Geometry: final body of the model. Coordinates: model frame, mm. A direction names the side the tool comes from. Give positions to 0.01 mm unless a question says otherwise; leave off trailing zeros. Loops run counter-clockwise (first coordinate to the right, second up) from the corner with the lowest first, then second, coordinate; pieces in that order, holes last. Notation, with made-up numbers: (6, 29.5) - (38, 29.5) arc R30 ccw to (38, 66.5) - close; hole circle Ø1 at (-22.5, 44). An arc over 180 degrees is marked (long way). Use CSV: the item, a comma, the result in double quotes. Start each with the question number.
```python
from build123d import *

# Parameters (mm, degrees)
SKETCH1_R            = 32.5
SKETCH1_R_2          = 17
BOSS_EXTRUDE1_DEPTH  = 6
SKETCH2_R            = 1.6
CUT_EXTRUDE1_DEPTH   = 6
LPATTERN1_COUNT      = 2
LPATTERN1_PITCH      = 36.8
LPATTERN1_COUNT_DIR2 = 2
LPATTERN1_PITCH_DIR2 = 36.8
SKETCH3_R            = 1.65
CUT_EXTRUDE2_DEPTH   = 10
CIRPATTERN1_COUNT    = 6
SKETCH6_W            = 10
SKETCH6_H            = 20
CUT_EXTRUDE4_DEPTH   = 10
SKETCH7_R            = 1.6
SKETCH7_R_2          = 1.5
CUT_EXTRUDE5_DEPTH   = 20
FILLET1_R            = 3.175
CUT_EXTRUDE6_START   = 3.1
SKETCH8_R            = 6
CUT_EXTRUDE6_DEPTH   = 20


with BuildPart() as part:
    # Sketch1 → Boss-Extrude1 (new body)
    with BuildSketch(Plane(origin=(0, 0, 0), x_dir=(1, 0, 0), z_dir=(0, 1, 0))):
        with BuildLine():
            Line((-42.5, -73.411966665), (-41.810700901, -77.192472856))
            ThreePointArc((-41.810700901, -77.192472856), (0, -112.069134335), (41.810700901, -77.192472856))
            Line((41.810700901, -77.192472856), (42.5, -73.411966665))
            Line((42.5, -73.411966665), (42.5, 36.289181897))
            ThreePointArc((42.5, 36.289181897), (39.241370505, 39.790319974), (35.695303931, 43))
            Line((35.695303931, 43), (-35.695303931, 43))
            ThreePointArc((-35.695303931, 43), (-39.241370505, 39.790319974), (-42.5, 36.289181897))
            Line((-42.5, 36.289181897), (-42.5, -73.411966665))
        make_face()
        with Locations(Location((0, 0, 0), (0, 0, 270))):
            Circle(SKETCH1_R, mode=Mode.SUBTRACT)
        with Locations(Location((0, -69.569134335, 0), (0, 0, 270))):
            Circle(SKETCH1_R_2, mode=Mode.SUBTRACT)
    extrude(amount=BOSS_EXTRUDE1_DEPTH)

    # Sketch2 → Cut-Extrude1 (cut)
    with BuildSketch(Plane(origin=(0, 6, 0), x_dir=(1, 0, 0), z_dir=(0, 1, 0))):
        with Locations(Location((18.4, -51.169134335, 0), (0, 0, 270))):
            Circle(SKETCH2_R)
    cut_extrude1 = extrude(amount=-CUT_EXTRUDE1_DEPTH, mode=Mode.SUBTRACT)

    # LPattern1: Cut-Extrude1 2 × 2
    with Locations(*[(-j * LPATTERN1_PITCH_DIR2, 0, i * LPATTERN1_PITCH) for i in range(LPATTERN1_COUNT) for j in range(LPATTERN1_COUNT_DIR2) if (i, j) != (0, 0)]):
        add(cut_extrude1, mode=Mode.SUBTRACT)

    # Sketch3 → Cut-Extrude2 (cut)
    with BuildSketch(Plane(origin=(0, 6, 0), x_dir=(1, 0, 0), z_dir=(0, 1, 0))):
        with Locations(Location((0, 38.5, 0), (0, 0, 270))):
            Circle(SKETCH3_R)
    cut_extrude2 = extrude(amount=-CUT_EXTRUDE2_DEPTH, mode=Mode.SUBTRACT)

    # CirPattern1: Cut-Extrude2 ×6 about axis
    cirpattern1_axis = Axis((0, 0, 0), (0, 1, 0))
    for i in range(1, CIRPATTERN1_COUNT):
        add(cut_extrude2.rotate(cirpattern1_axis, i * 360 / CIRPATTERN1_COUNT), mode=Mode.SUBTRACT)

    # Sketch6 → Cut-Extrude4 (cut)
    with BuildSketch(Plane(origin=(0, 6, 0), x_dir=(1, 0, 0), z_dir=(0, 1, 0))):
        with Locations((0, -112.069134335)):
            Rectangle(SKETCH6_W, SKETCH6_H)
    extrude(amount=-CUT_EXTRUDE4_DEPTH, mode=Mode.SUBTRACT)

    # Sketch7 → Cut-Extrude5 (cut)
    with BuildSketch(Plane(origin=(0, 0, 0), x_dir=(1, 0, 0), z_dir=(0, 1, 0))):
        with Locations(Location((-27.5, -34.784567168, 0), (0, 0, 270))):
            Circle(SKETCH7_R)
        with Locations(Location((-25.829771931, -81.613754795, 0), (0, 0, 270))):
            Circle(SKETCH7_R_2)
        with Locations(Location((25.829771931, -81.613754795, 0), (0, 0, 270))):
            Circle(SKETCH7_R_2)
        with Locations(Location((27.5, -34.784567168, 0), (0, 0, 270))):
            Circle(SKETCH7_R)
    extrude(amount=CUT_EXTRUDE5_DEPTH, mode=Mode.SUBTRACT)

    # Fillet1
    fillet1_edges = [part.edges().sort_by_distance(p)[0] for p in [
        (-5, 3, 102.069134335),
        (5, 3, 102.069134335),
    ]]
    fillet(fillet1_edges, radius=FILLET1_R)

    # Sketch8 → Cut-Extrude6 (cut)
    with BuildSketch(Plane(origin=(0, 0, 0), x_dir=(1, 0, 0), z_dir=(0, 1, 0)).offset(CUT_EXTRUDE6_START)):
        with Locations(Location((-28.5, 29, 0), (0, 0, 270))):
            Circle(SKETCH8_R)
        with Locations((-32.5, -26.784567168)):
            Circle(SKETCH8_R)
        with Locations((32.5, -26.784567168)):
            Circle(SKETCH8_R)
        with Locations(Location((28.5, 29, 0), (0, 0, 270))):
            Circle(SKETCH8_R)
    extrude(amount=CUT_EXTRUDE6_DEPTH, mode=Mode.SUBTRACT)


solid = part.part
```
Item 1: Section C-C (y = 1.65). Give the number of separate pieces and of enclosed holes in the cut face, plus the area to 3 significant figures.
Item 2: Ray query, probe 1 along X at (y, z) = (4.45, 35); probe 2 along Z at (x, y) = (3, 1.05); probe 3 along X at (y, z) = (2.3, 38.5). Return the intervals inside material, ascending.
Item 3: Section B-B (x = -11.5). Output: boundary loops of the cut face in (y, z), plus the area to 3 significant figures.
Item 4: Mould query, pull axis X, two halves, no side actions, for faces 1 (the flat face through (-42.5, 3, 18)), 2 (the flat face through (42.15, 2.96, 75.33)), 3 (the cylindrical face through (-32.15, 4.53, -33.76)), 4 (the cylindrical face through (9.76, 2.96, 31)). Classes: pulls with the +X half, pulls with the -X half, needs draft (parallel to the pull), parting line crosses it, or undercut.
Item 5: Reachability of faces 5 (the cylindrical face through (-18.33, 3.04, 86.37)), 6 (the cylindrical face through (4.045, 2.958, 102.975)) from +Z, -Z, +X, -X, +Y, -Y: full face, straight path, thin tool, end or side. Return the list, or none.
Item 6: Pin query (flat end, axial travel): pin 1 Ø9.5 at (x, z) = (-34, 27) entering from +Y; pin 2 Ø1.8 at (y, z) = (2, 109) entering from -X; pin 3 Ø1.5 at (x, y) = (30.5, 5.5) entering from +Z; pin 4 Ø2.5 at (x, z) = (33.34, 19.25) entering from -Y. Return the tip coordinate at first contact, or that it passes through.
Item 7: Section A-A (z = -29). Output: boundary loops of the cut face in (x, y).
Item 8: Section D-D (z = 10.5). Output: boundary loops of the cut face in (x, y).
Outcome:
1,separate pieces,"1"
1,enclosed holes,"16"
1,area,"7,930 mm2"
2,probe 1,"x = -42.5 to -29.09, -25.91 to 25.91, 29.09 to 42.5"
2,probe 2,"z = -43 to -32.36, 32.36 to 52.84, 86.3 to 102.29"
2,probe 3,"x = -42.5 to -1.65, 1.65 to 42.5"
3,outline,"(0, -43) - (6, -43) - (6, -30.4) - (0, -30.4) - close; (0, 30.4) - (6, 30.4) - (6, 57.05) - (0, 57.05) - close; (0, 82.09) - (6, 82.09) - (6, 110.48) - (0, 110.48) - close"
3,area,"406 mm2"
4,face 1,"pulls with the -X half"
4,face 2,"pulls with the +X half"
4,face 3,"undercut"
4,face 4,"undercut"
5,face 5,"+Y, -Y"
5,face 6,"+Z, +Y, -Y"
6,pin 1,"stops at y = 6"
6,pin 2,"stops at x = -17.93"
6,pin 3,"stops at z = 99.92"
6,pin 4,"passes through"
7,outline,"(-42.5, 0) - (-14.67, 0) - (-14.67, 6) - (-22.5, 6) - (-22.5, 3.1) - (-34.5, 3.1) - (-34.5, 6) - (-42.5, 6) - close; (14.67, 0) - (42.5, 0) - (42.5, 6) - (34.5, 6) - (34.5, 3.1) - (22.5, 3.1) - (22.5, 6) - (14.67, 6) - close"
8,outline,"(-42.5, 0) - (-30.76, 0) - (-30.76, 6) - (-42.5, 6) - close; (30.76, 0) - (42.5, 0) - (42.5, 6) - (30.76, 6) - close"
